from build123d import *

# Parameters (mm, degrees)
SKETCH1_W            = 65.5
SKETCH1_H            = 65.5
BOSS_EXTRUDE1_DEPTH  = 3
SKETCH5_R            = 2.55
CUT_EXTRUDE5_DEPTH   = 4
LPATTERN2_COUNT      = 5
LPATTERN2_PITCH      = 10
LPATTERN2_COUNT_DIR2 = 2
LPATTERN2_PITCH_DIR2 = 39.7
SKETCH7_R            = 2.55
CUT_EXTRUDE6_DEPTH   = 4
SKETCH8_R            = 2.55
CUT_EXTRUDE7_DEPTH   = 4
CIRPATTERN1_COUNT    = 4
CUT_EXTRUDE4_START   = -1
SKETCH3_R            = 3.6
CUT_EXTRUDE4_DEPTH   = 5
LPATTERN1_COUNT      = 3
LPATTERN1_PITCH      = 20
CUT_EXTRUDE8_DEPTH   = 4
LPATTERN3_COUNT      = 3
LPATTERN3_PITCH      = 19.85
LPATTERN3_COUNT_DIR2 = 2
LPATTERN3_PITCH_DIR2 = 55.4
CUT_EXTRUDE9_DEPTH   = 4
LPATTERN4_COUNT      = 2
LPATTERN4_PITCH      = 40
FILLET1_R            = 3


with BuildPart() as part:
    # Sketch1 → Boss-Extrude1 (new body)
    with BuildSketch(Plane(origin=(0, 0, 0), x_dir=(1, 0, 0), z_dir=(0, 1, 0))):
        Rectangle(SKETCH1_W, SKETCH1_H)
    extrude(amount=BOSS_EXTRUDE1_DEPTH)

    # Sketch5 → Cut-Extrude5 (cut, through all)
    with BuildSketch(Plane(origin=(0, 0, 0), x_dir=(1, 0, 0), z_dir=(0, 1, 0))):
        with Locations((-19.85, 20)):
            Circle(SKETCH5_R)
    cut_extrude5 = extrude(amount=CUT_EXTRUDE5_DEPTH, mode=Mode.SUBTRACT)

    # LPattern2: Cut-Extrude5 5 × 2
    with Locations(*[(j * LPATTERN2_PITCH_DIR2, 0, i * LPATTERN2_PITCH) for i in range(LPATTERN2_COUNT) for j in range(LPATTERN2_COUNT_DIR2) if (i, j) != (0, 0)]):
        add(cut_extrude5, mode=Mode.SUBTRACT)

    # Sketch7 → Cut-Extrude6 (cut, through all)
    with BuildSketch(Plane(origin=(0, 0, 0), x_dir=(1, 0, 0), z_dir=(0, 1, 0))):
        Circle(SKETCH7_R)
    extrude(amount=CUT_EXTRUDE6_DEPTH, mode=Mode.SUBTRACT)

    # Sketch8 → Cut-Extrude7 (cut, through all)
    with BuildSketch(Plane(origin=(0, 0, 0), x_dir=(1, 0, 0), z_dir=(0, 1, 0))):
        with Locations((0, 10)):
            Circle(SKETCH8_R)
    cut_extrude7 = extrude(amount=CUT_EXTRUDE7_DEPTH, mode=Mode.SUBTRACT)

    # CirPattern1: Cut-Extrude7 ×4 about axis
    cirpattern1_axis = Axis((0, 0, 0), (0, 1, 0))
    for i in range(1, CIRPATTERN1_COUNT):
        add(cut_extrude7.rotate(cirpattern1_axis, i * 360 / CIRPATTERN1_COUNT), mode=Mode.SUBTRACT)

    # Sketch3 → Cut-Extrude4 (cut)
    with BuildSketch(Plane(origin=(0, 0, 0), x_dir=(1, 0, 0), z_dir=(0, 1, 0)).offset(CUT_EXTRUDE4_START)):
        with Locations((-19.85, 20)):
            Circle(SKETCH3_R)
    cut_extrude4 = extrude(amount=CUT_EXTRUDE4_DEPTH, mode=Mode.SUBTRACT)

    # LPattern1: Cut-Extrude4 ×3
    with Locations(*[(0, 0, i * LPATTERN1_PITCH) for i in range(1, LPATTERN1_COUNT)]):
        add(cut_extrude4, mode=Mode.SUBTRACT)

    # Sketch9 → Cut-Extrude8 (cut, through all)
    with BuildSketch(Plane(origin=(0, 0, 0), x_dir=(1, 0, 0), z_dir=(0, 1, 0))):
        with BuildLine():
            Line((-23.1, 29.2), (-16.6, 29.2))
            ThreePointArc((-16.6, 29.2), (-15.1, 27.7), (-16.6, 26.2))
            Line((-16.6, 26.2), (-23.1, 26.2))
            ThreePointArc((-23.1, 26.2), (-24.6, 27.7), (-23.1, 29.2))
        make_face()
    cut_extrude8 = extrude(amount=CUT_EXTRUDE8_DEPTH, mode=Mode.SUBTRACT)

    # LPattern3: Cut-Extrude8 3 × 2
    with Locations(*[(i * LPATTERN3_PITCH, 0, j * LPATTERN3_PITCH_DIR2) for i in range(LPATTERN3_COUNT) for j in range(LPATTERN3_COUNT_DIR2) if (i, j) != (0, 0)]):
        add(cut_extrude8, mode=Mode.SUBTRACT)

    # Sketch10 → Cut-Extrude9 (cut, through all)
    with BuildSketch(Plane(origin=(0, 0, 0), x_dir=(1, 0, 0), z_dir=(0, 1, 0))):
        with BuildLine():
            Line((-10.05, 22.5), (10.05, 22.5))
            ThreePointArc((10.05, 22.5), (12.55, 20), (10.05, 17.5))
            Line((10.05, 17.5), (-10.05, 17.5))
            ThreePointArc((-10.05, 17.5), (-12.55, 20), (-10.05, 22.5))
        make_face()
    cut_extrude9 = extrude(amount=CUT_EXTRUDE9_DEPTH, mode=Mode.SUBTRACT)

    # LPattern4: Cut-Extrude9 ×2
    with Locations(*[(0, 0, i * LPATTERN4_PITCH) for i in range(1, LPATTERN4_COUNT)]):
        add(cut_extrude9, mode=Mode.SUBTRACT)

    # Fillet1
    fillet1_edges = [part.edges().sort_by_distance(p)[0] for p in [
        (32.75, 1.5, 32.75),
        (-32.75, 1.5, 32.75),
        (-32.75, 1.5, -32.75),
        (32.75, 1.5, -32.75),
    ]]
    fillet(fillet1_edges, radius=FILLET1_R)


solid = part.part
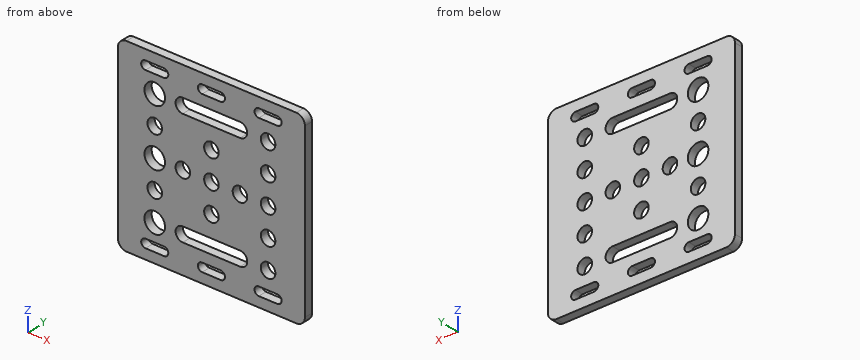
Read the model definition and answer for the solid it produces. Units are mm, in the model's axes. Round coordinates to 2 decimals unless told otherwise and drop trailing zeros. Order: outer loops, then holes, each group sorted by start corner. A loop starts at its lowest first (then second) coordinate and runs counter-clockwise, first axis right, second up.
1) The part is cut by section A-A on z = -20. Write down the section's boundary in (x, y), plus the area to 3 significant figures.
2) The part is cut by section B-B on x = 0. Give the number of separate pieces and of enclosed holes in the cut face, plus the area to 3 significant figures.
3) Straight lines are drawn through the part: L1, parallel to Z at x = -7, y = 2.1; L2, parallel to Z at x = 23, y = 2.4; L3, parallel to Z at x = -4, y = 1.7. For each, find the intervals that lie inside material, in ascending order.
4) The part is cut by section C-C on z = 27.7. Write down the section's boundary in (x, y).
Resolved:
1. outline: (-32.75, 0) - (-23.45, 0) - (-23.45, 3) - (-32.75, 3) - close; (-16.25, 0) - (-12.55, 0) - (-12.55, 3) - (-16.25, 3) - close; (12.55, 0) - (17.3, 0) - (17.3, 3) - (12.55, 3) - close; (22.4, 0) - (32.75, 0) - (32.75, 3) - (22.4, 3) - close
1. area: 84.3 mm2
2. separate pieces: 8
2. enclosed holes: 0
2. area: 103 mm2
3. L1: z = -32.75 to -22.5, -17.5 to 17.5, 22.5 to 32.75
3. L2: z = -32.75 to -29.2, -26.2 to 26.2, 29.2 to 32.75
3. L3: z = -32.75 to -29, -26.4 to -22.5, -17.5 to 17.5, 22.5 to 26.4, 29 to 32.75
4. outline: (-32.75, 0) - (-24.6, 0) - (-24.6, 3) - (-32.75, 3) - close; (-15.1, 0) - (-4.75, 0) - (-4.75, 3) - (-15.1, 3) - close; (4.75, 0) - (15.1, 0) - (15.1, 3) - (4.75, 3) - close; (24.6, 0) - (32.75, 0) - (32.75, 3) - (24.6, 3) - close
